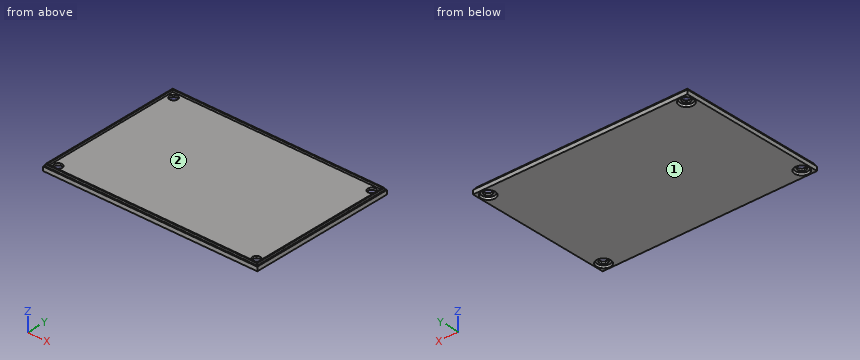
from build123d import *

# Parameters (mm, degrees)
F0_W     = 106.5
F0_H     = 72.5
F1_DEPTH = 2
F2_R     = 2
F3_DEPTH = 2
F4_R     = 3.5
F5_DEPTH = 1
F5_TAPER = 20
F6_W     = 105.25
F6_H     = 71.125
F6_W_2   = 104.25
F6_H_2   = 70.125
F7_DEPTH = 1


with BuildPart() as f1:
    # F0 (on Top) → F1 (new body)
    with BuildSketch(Plane.XY):
        with Locations((-53.25, 36.25)):
            Rectangle(F0_W, F0_H)
    extrude(amount=F1_DEPTH)

    # F2 (on face) → F3 (cut, through all)
    with BuildSketch(Plane.XY.offset(2)):
        with Locations((-102.5, 68.5)):
            Circle(F2_R)
        with Locations((-4, 68.5)):
            Circle(F2_R)
        with Locations((-4, 4)):
            Circle(F2_R)
        with Locations((-102.5, 4)):
            Circle(F2_R)
    extrude(amount=-F3_DEPTH, mode=Mode.SUBTRACT)

    # F4 (on face) → F5 (cut)
    with BuildSketch(Plane(origin=(0, 0, 0), x_dir=(1, 0, 0), z_dir=(0, 0, -1))):
        with Locations((-102.5, -4)):
            Circle(F4_R)
        with Locations((-4, -4)):
            Circle(F4_R)
        with Locations((-102.5, -68.5)):
            Circle(F4_R)
        with Locations((-4, -68.5)):
            Circle(F4_R)
    extrude(amount=-F5_DEPTH, taper=F5_TAPER, mode=Mode.SUBTRACT)

    # F6 (on face) → F7 (join)
    with BuildSketch(Plane.XY.offset(2)):
        with Locations((-53.25, 36.1875)):
            Rectangle(F6_W, F6_H)
        with Locations((-53.25, 36.1875)):
            Rectangle(F6_W_2, F6_H_2, mode=Mode.SUBTRACT)
    extrude(amount=F7_DEPTH)


solid = f1.part
Geometry: final body of the model. Coordinates: model frame, mm. Face numbers are marked on the shaded views. Give positions to 0.01 mm unless a question says otherwise; leave off trailing zeros. Write each loop counter-clockwise with the first axis right and the second up, starting at its lowest first coordinate (ties: lowest second). Pieces come first, ordered by that corner, then holes. Notation, with made-up numbers: (49.5, 64) -> (104.5, 64) arc R17 cw to (104.5, 71) -> close; hole circle Ø10 at (17, 1). An arc over 180 degrees is marked (long way). Answer in a Markdown table with one row per item.
(1) Section query D-D on x = -58. Return loops of the section in (y, z) (3 decimals), then the cut area to 3 significant figures.
Answers below:
| item | result |
|---|---|
| outline | (0, 0) -> (72.5, 0) -> (72.5, 2) -> (71.75, 2) -> (71.75, 3) -> (71.25, 3) -> (71.25, 2) -> (1.125, 2) -> (1.125, 3) -> (0.625, 3) -> (0.625, 2) -> (0, 2) -> close |
| area | 146 mm^2 |
(2) Section query A-A on x = -102.5. Return loops of the section in (y, z) (3 decimals), then the cut area to 3 significant figures.
Answers below:
| item | result |
|---|---|
| outline | (0, 0) -> (0.5, 0) -> (0.864, 1) -> (2, 1) -> (2, 2) -> (1.125, 2) -> (1.125, 3) -> (0.625, 3) -> (0.625, 2) -> (0, 2) -> close; (6, 1) -> (7.136, 1) -> (7.5, 0) -> (65, 0) -> (65.364, 1) -> (66.5, 1) -> (66.5, 2) -> (6, 2) -> close; (70.5, 1) -> (71.636, 1) -> (72, 0) -> (72.5, 0) -> (72.5, 2) -> (71.75, 2) -> (71.75, 3) -> (71.25, 3) -> (71.25, 2) -> (70.5, 2) -> close |
| area | 125 mm^2 |
(3) Ray query, line 1 along Y through (x, z) = (-4, 1.65); line 2 along X through (y, z) = (13, 2.4) (3 decimals); line 3 along Y through (x, z) = (-90.5, 2.8) (3 decimals). Return the intervals inside material, ascending. Write a range as [from, to].
Answers below:
| item | result |
|---|---|
| line 1 | [0, 2], [6, 66.5], [70.5, 72.5] |
| line 2 | [-105.875, -105.375], [-1.125, -0.625] |
| line 3 | [0.625, 1.125], [71.25, 71.75] |
(4) Section query C-C on y = 4. State how many separate pieces and enclosed holes the cut face has, then the cut area to 3 significant figures.
Answers below:
| item | result |
|---|---|
| separate pieces | 3 |
| enclosed holes | 0 |
| area | 193 mm^2 |
(5) Draft query along Y for the marked faces 1 and 2. Return one class per face: +Y half, -Y half, draft (parallel to the pull), parting line (faces both ways), or undercut.
Answers below:
| item | result |
|---|---|
| face 1 | draft |
| face 2 | undercut |
(6) Pin query (flat end, axial travel): pin 1 (1.1 mm diameter, centred on x = -32, z = 2.5, fed in from +Y); pin 2 (8 mm diameter, centred on x = -34, y = 40.5, fed in from +Z); pin 3 (3 mm diameter, centred on x = -103, y = 2.5, fed in from -Z). Return the tip coordinate at first contact, or that it passes through.
Answers below:
| item | result |
|---|---|
| pin 1 | y = 72.5 |
| pin 2 | z = 2 |
| pin 3 | z = 1 |
(7) Section query B-B on y = 40. Return loops of the section in (x, z) (3 decimals), then the cut area to 3 significant figures.
Answers below:
| item | result |
|---|---|
| outline | (-106.5, 0) -> (0, 0) -> (0, 2) -> (-0.625, 2) -> (-0.625, 3) -> (-1.125, 3) -> (-1.125, 2) -> (-105.375, 2) -> (-105.375, 3) -> (-105.875, 3) -> (-105.875, 2) -> (-106.5, 2) -> close |
| area | 214 mm^2 |
